Autodesk Inventor part; units mm, degrees
ref_plane "YZ Plane" through (0, 0, 0) normal (1, 0, 0) x (0, 1, 0)
ref_plane "XZ Plane" through (0, 0, 0) normal (0, 1, 0) x (-1, 0, 0)
ref_plane "XY Plane" through (0, 0, 0) normal (0, 0, 1) x (1, 0, 0)
sketch "Sketch1" plane through (0, 0, 0) normal (0, 1, 0) x (-1, 0, 0)
  line L0 (32, -0.4496) -> (0, -0.4496)
  line L1 (-80.1396, -91.6786) -> (-80.1396, -109.8686)
  line L2 (37, -56.2289) -> (-80, -56.2289)
  line L3 (-43.5, -0.4496) -> (-75, -0.4496)
  line L4 (37.1396, -109.8686) -> (37.1396, -91.6786)
  arc A0 (-60, -65.8686) -> (-58, -67.8686) centre (-58, -65.8686) ccw
  line L5 (15, -67.8686) -> (-58, -67.8686)
  arc A1 (15, -67.8686) -> (17, -65.8686) centre (15, -65.8686) ccw
  line L6 (17, -50.7793) -> (17, -65.8686)
  arc A2 (27, -35.7793) -> (25, -33.7793) centre (25, -35.7793) ccw
  line L7 (-6, -33.7793) -> (25, -33.7793)
  arc A3 (-6, -33.7793) -> (-8, -35.7793) centre (-6, -35.7793) ccw
  line L8 (-8, -36.7793) -> (-8, -35.7793)
  arc A4 (-10, -38.7793) -> (-8, -36.7793) centre (-10, -36.7793) ccw
  arc A5 (-35, -36.7793) -> (-33, -38.7793) centre (-33, -36.7793) ccw
  line L9 (-35, -35.7793) -> (-35, -36.7793)
  arc A6 (-35, -35.7793) -> (-37, -33.7793) centre (-37, -35.7793) ccw
  line L10 (-68, -33.7793) -> (-37, -33.7793)
  arc A7 (-68, -33.7793) -> (-70, -35.7793) centre (-68, -35.7793) ccw
  line L11 (-70, -46.7793) -> (-70, -35.7793)
  line L12 (-27.5, -31.2793) -> (-27.5, -8.2793)
  line L13 (-15.5, -31.2793) -> (-27.5, -31.2793)
  line L14 (-15.5, -8.2793) -> (-15.5, -31.2793)
  line L15 (-27.5, -8.2793) -> (-15.5, -8.2793)
  circle A8 centre (-21.5, -5.7793) radius 1.25
  circle A9 centre (-21.5, -33.7793) radius 1.25
  arc A10 (-1.04, -19.5193) -> (0.96, -21.5193) centre (0.96, -19.5193) ccw
  line L16 (11.96, -21.5193) -> (0.96, -21.5193)
  arc A11 (0.96, -9.5193) -> (-1.04, -11.5193) centre (0.96, -11.5193) ccw
  line L17 (-1.04, -19.5193) -> (-1.04, -11.5193)
  arc A12 (11.96, -21.5193) -> (13.96, -19.5193) centre (11.96, -19.5193) ccw
  line L18 (13.96, -11.5193) -> (13.96, -19.5193)
  arc A13 (13.96, -11.5193) -> (11.96, -9.5193) centre (11.96, -11.5193) ccw
  line L19 (0.96, -9.5193) -> (11.96, -9.5193)
  arc A14 (-43.96, -21.5193) -> (-41.96, -19.5193) centre (-43.96, -19.5193) ccw
  line L20 (-41.96, -11.5193) -> (-41.96, -19.5193)
  arc A15 (-56.96, -19.5193) -> (-54.96, -21.5193) centre (-54.96, -19.5193) ccw
  line L21 (-43.96, -21.5193) -> (-54.96, -21.5193)
  arc A16 (-41.96, -11.5193) -> (-43.96, -9.5193) centre (-43.96, -11.5193) ccw
  line L22 (-54.96, -9.5193) -> (-43.96, -9.5193)
  arc A17 (-54.96, -9.5193) -> (-56.96, -11.5193) centre (-54.96, -11.5193) ccw
  line L23 (-56.96, -19.5193) -> (-56.96, -11.5193)
  arc A18 (25, -48.7793) -> (27, -46.7793) centre (25, -46.7793) ccw
  line L24 (27, -35.7793) -> (27, -46.7793)
  arc A19 (19, -48.7793) -> (17, -50.7793) centre (19, -50.7793) ccw
  arc A20 (-60, -50.7793) -> (-62, -48.7793) centre (-62, -50.7793) ccw
  line L25 (-60, -65.8686) -> (-60, -50.7793)
  arc A21 (-70, -46.7793) -> (-68, -48.7793) centre (-68, -46.7793) ccw
  line L26 (-62, -48.7793) -> (-68, -48.7793)
  line L27 (25, -48.7793) -> (19, -48.7793)
  line L28 (-33, -38.7793) -> (-10, -38.7793)
  circle A22 centre (-59, 25.095) radius 1.55
  circle A23 centre (16, 25.095) radius 1.55
  circle A24 centre (-89.6843, -101.7736) radius 1.55
  circle A25 centre (46.6843, -101.7736) radius 1.55
  arc A26 (-80, -88.6786) -> (-79, -89.6786) centre (-79, -88.6786) ccw
  arc A27 (36, -89.6786) -> (37, -88.6786) centre (36, -88.6786) ccw
  line L29 (35.94, -89.6786) -> (36, -89.6786)
  arc A28 (55.7793, -92.6786) -> (54.7793, -91.6786) centre (54.7793, -92.6786) ccw
  arc A29 (54.7793, -109.8686) -> (55.7793, -108.8686) centre (54.7793, -108.8686) ccw
  line L30 (54.7793, -109.8686) -> (-97.7793, -109.8686)
  arc A30 (-98.7793, -108.8686) -> (-97.7793, -109.8686) centre (-97.7793, -108.8686) ccw
  arc A31 (-97.7793, -91.6786) -> (-98.7793, -92.6786) centre (-97.7793, -92.6786) ccw
  line L31 (-97.7793, -91.6786) -> (-78.94, -91.6786)
  arc A32 (1, 33.19) -> (0, 32.19) centre (1, 32.19) ccw
  arc A33 (32, 32.19) -> (31, 33.19) centre (31, 32.19) ccw
  arc A34 (-74, 33.19) -> (-75, 32.19) centre (-74, 32.19) ccw
  arc A35 (-43.5, 32.19) -> (-44.5, 33.19) centre (-44.5, 32.19) ccw
  line L32 (-43.5, 32.19) -> (-43.5, -1.6493)
  line L33 (-74, 33.19) -> (-44.5, 33.19)
  line L34 (-75, -1.6493) -> (-75, 32.19)
  line L35 (-75, -1.6493) -> (-80, -1.6493)
  line L36 (-80, -88.6786) -> (-80, -1.6493)
  line L37 (1, 33.19) -> (31, 33.19)
  line L38 (32, 32.19) -> (32, -1.6493)
  line L39 (37, -1.6493) -> (32, -1.6493)
  line L40 (0, -1.6493) -> (0, 32.19)
  line L41 (0, -1.6493) -> (-43.5, -1.6493)
  line L42 (37, -1.6493) -> (37, -88.6786)
  line L43 (-98.7793, -108.8686) -> (-98.7793, -92.6786)
  line L44 (55.7793, -92.6786) -> (55.7793, -108.8686)
  line L45 (35.94, -91.6786) -> (54.7793, -91.6786)
  line L46 (35.94, -91.6786) -> (35.94, -89.6786)
  line L47 (-79, -89.6786) -> (-78.94, -89.6786)
  line L48 (-78.94, -89.6786) -> (-78.94, -91.6786)
  line L49 (-80.5893, -109.8686) -> (-80.5893, -91.6786)
  line L50 (37.5893, -91.6786) -> (37.5893, -109.8686)
  line L51 (-79.69, -91.6786) -> (-79.69, -109.8686)
  line L52 (36.69, -109.8686) -> (36.69, -91.6786)
  line L53 (-75, 0) -> (-43.5, 0)
  line L54 (37, -56.6786) -> (17, -56.6786)
  line L55 (-60, -56.6786) -> (-80, -56.6786)
  line L56 (-43.5, -0.8993) -> (-75, -0.8993)
  line L57 (17, -55.7793) -> (37, -55.7793)
  line L58 (-80, -55.7793) -> (-60, -55.7793)
  line L59 (32, -0.8993) -> (0, -0.8993)
  line L60 (0, 0) -> (32, 0)
  point P0 (0, 0)
extrude "Plate1" add sketch "Sketch1" against normal blind 1.5 contours L38 L59 L40 L0 | L0 L40 L60 L38 | L60 L40 A32 L37 A33 L38 | L38 L39 L42 L57 L6 A19 L27 A18 L24 A2 L7 A3 L8 A4 L28 A5 L9 A6 L10 A7 L11 A21 L26 A20 L25 L58 L36 L35 L34 L56 L32 L41 L40 L59 | L42 L2 L6 L57 | L56 L34 L3 L32 | L42 L54 L6 L2 | L3 L34 L53 L32 | L42 A27 L29 L46 L45 L52 L30 L51 L31 L48 L47 A26 L36 L55 L25 A0 L5 A1 L6 L54 | L53 L34 A34 L33 A35 L32 | L25 L55 L36 L2 | L2 L36 L58 L25 | L45 L4 L30 L52 | L45 L50 L30 L4 | L45 A28 L44 A29 L30 L50 | L30 L1 L31 L51 | L30 L49 L31 L1 | L30 A30 L43 A31 L31 L49
equation "\"d0\" = Thickness"
equation "\"BendReliefWidth\" = Thickness"
equation "\"BendReliefDepth\" = 0.5 * Thickness"
equation "\"CornerReliefSize\" = 4 * Thickness"
equation "\"MinimumRemnant\" = 2 * Thickness"
equation "\"TransitionRadius\" = BendRadius"
equation "\"JacobiRadiusSize\" = BendRadius"
equation "\"GapSize\" = Thickness"
properties part number "body_top_frame2_cam" material "Aluminum 6061-AHC"
Could you check a few things on this model? Use its own coordinates, in mm. Coordinates: 2 decimals unless noted, no trailing zeros. Order: outer loops, then holes, each group sorted by start corner. A loop starts at its lowest first (then second) coordinate and runs counter-clockwise, first axis right, second up.
Q1. Please list where these lines run through material, in increasing order: L1, parallel to X at y = -0.5, z = -36.5; L2, parallel to X at y = -1.05, z = -14; L3, parallel to Z at x = 53, y = -1.
Q2. Suppose I cut it at C-C on x = -34. Please give me the cut outline in (y, z), and give its area (3 significant figures).
Q3. Suppose I cut it at B-B on z = 14.5. Please give me the cut outline in (x, y), and give its area (4 significant figures).
Q4. Suppose I cut it at A-A on x = 50. Please give me the cut outline in (y, z), and give its area (3 significant figures).
Q5. Suppose I cut it at D-D on y = -1.05. Give the number of separate pieces and of enclosed holes in the cut face, and give its area (3 significant figures).
Q6. Will these pins go through, and if not, where does the flat tip stop? pin 1 (0.8 mm diameter, centred on y = -1, z = -36.5, fed in from +X); pin 2 (0.8 mm diameter, centred on y = -0.5, z = -40, fed in from -X).
Answer:
1. L1: x = -37 to -27, 8 to 35, 70 to 80
1. L2: x = -37 to -13.96, 1.04 to 15.5, 27.5 to 41.96, 56.96 to 80
1. L3: z = -109.87 to -67.87, -33.78 to -21.52, -9.52 to 33.19
2. outline: (-1.5, -109.87) - (0, -109.87) - (0, -1.65) - (-1.5, -1.65) - close
2. area: 162 mm2
3. outline: (-32, -1.5) - (0, -1.5) - (0, 0) - (-32, 0) - close; (43.5, -1.5) - (75, -1.5) - (75, 0) - (43.5, 0) - close
3. area: 95.25 mm2
4. outline: (-1.5, -109.87) - (0, -109.87) - (0, -67.87) - (-1.5, -67.87) - close; (-1.5, -33.78) - (0, -33.78) - (0, -21.52) - (-1.5, -21.52) - close; (-1.5, -9.52) - (0, -9.52) - (0, 33.19) - (-1.5, 33.19) - close
4. area: 145 mm2
5. separate pieces: 1
5. enclosed holes: 10
5. area: 12,100 mm2
6. pin 1: stops at x = 80
6. pin 2: stops at x = -37
